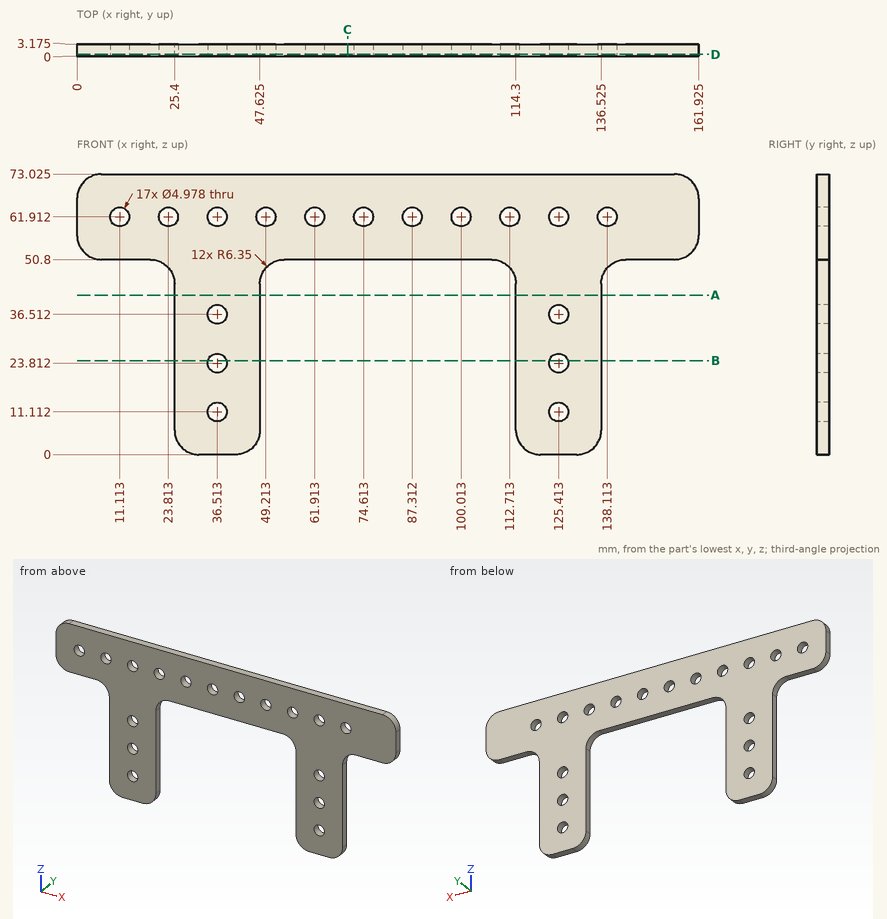
Job drawing, mm, ordinate dimensions from the low corner. One solid piece. Coordinates: 2 decimals unless noted, no trailing zeros. Order: outer loops, then holes, each group sorted by start corner. A loop starts at its lowest first (then second) coordinate and runs counter-clockwise, first axis right, second up. Notation, with made-up numbers: (20.25, 3) - (76.25, 3) arc R19 ccw to (76.25, 30) - close; hole circle Ø3 at (-16, 24.5). An arc over 180 degrees is marked (long way). Use CSV: the item, a comma, the result in double quotes.
Item 1: Probe probe 1 along X at (y, z) = (1.2, 37.5) (1 decimal); probe 2 along X at (y, z) = (1.2, 18.5) (1 decimal); probe 3 along X at (y, z) = (0.95, 25) (1 decimal). List the from-to ranges inside material, lowest first.
Solved:
probe 1,"x = 25.4 to 34.2, 38.8 to 47.6, 114.3 to 123.1, 127.7 to 136.5"
probe 2,"x = 25.4 to 47.6, 114.3 to 136.5"
probe 3,"x = 25.4 to 34.3, 38.7 to 47.6, 114.3 to 123.2, 127.6 to 136.5"
Item 2: Drop flat-ended pins along their axis: P1, Ø1, axis at x = 33, y = 0.5, coming from the -Z side; P2, Ø1, axis at y = 2.5, z = 29, coming from the +X side (1 decimal); P3, Ø1, axis at y = 2, z = 34.5, coming from the -X side; P4, Ø4.5, axis at x = 138.11, z = 61.91, coming from the +Y side. Give the stop position or say it passes through.
Solved:
P1,"stops at z = 0"
P2,"stops at x = 136.5"
P3,"stops at x = 25.4"
P4,"passes through"
Item 3: Saw through at D-D on y = 0.5. Give the number of separate pieces and of enclosed holes in the cut face, and give its area (3 significant figures).
Solved:
separate pieces,"1"
enclosed holes,"17"
area,"5,490 mm²"
Item 4: Saw through at B-B on z = 24.5. Give the cut face in (x, y) (1 decimal).
Solved:
outline,"(25.4, 0) - (34.1, 0) - (34.1, 3.2) - (25.4, 3.2) - close; (38.9, 0) - (47.6, 0) - (47.6, 3.2) - (38.9, 3.2) - close; (114.3, 0) - (123, 0) - (123, 3.2) - (114.3, 3.2) - close; (127.8, 0) - (136.5, 0) - (136.5, 3.2) - (127.8, 3.2) - close"
Item 5: Saw through at C-C on x = 70.5. Give the cut face in (y, z) (1 decimal).
Solved:
outline,"(0, 50.8) - (3.2, 50.8) - (3.2, 73) - (0, 73) - close"
Item 6: Saw through at A-A on z = 41.5. Give the cut face in (x, y) (1 decimal), and give its area (3 significant figures).
Solved:
outline,"(25.4, 0) - (47.6, 0) - (47.6, 3.2) - (25.4, 3.2) - close; (114.3, 0) - (136.5, 0) - (136.5, 3.2) - (114.3, 3.2) - close"
area,"141 mm²"
